```python
from build123d import *

# Parameters (mm, degrees)
SKETCH1_R                    = 211.670411635
SKETCH1_R_2                  = 6.985
SKETCH1_R_3                  = 6.6294
SKETCH1_R_4                  = 5.8928
SKETCH1_R_5                  = 4.2291
SKETCH1_R_6                  = 5.461
SKETCH1_R_7                  = 5.7531
SKETCH1_R_8                  = 5.4991
SKETCH1_R_9                  = 7.7978
SKETCH1_R_10                 = 6.6421
SKETCH1_R_11                 = 4.6228
SKETCH1_R_12                 = 5.9182
BOSS_EXTRUDE1_DEPTH          = 6
SKETCH2_R                    = 87.5
CUT_EXTRUDE1_DEPTH           = 300.4072917
F_3_8_0_375_DIAMETER_HOLE1_D = 9.525
CIRPATTERN1_COUNT            = 4


with BuildPart() as part:
    # Sketch1 → Boss-Extrude1 (new body)
    with BuildSketch(Plane.XY):
        Circle(SKETCH1_R)
        with Locations((160.80232, -67.72402)):
            Circle(SKETCH1_R_2, mode=Mode.SUBTRACT)
        with Locations((129.93116, -131.74726)):
            Circle(SKETCH1_R_3, mode=Mode.SUBTRACT)
        with Locations((88.98382, -143.60906)):
            Circle(SKETCH1_R_4, mode=Mode.SUBTRACT)
        with Locations((51.13274, -156.81706)):
            Circle(SKETCH1_R_5, mode=Mode.SUBTRACT)
        with Locations((-44.93006, -170.61434)):
            Circle(SKETCH1_R_6, mode=Mode.SUBTRACT)
        with Locations((-97.40392, -154.3431)):
            Circle(SKETCH1_R_7, mode=Mode.SUBTRACT)
        with Locations((-174.33036, -9.32688)):
            Circle(SKETCH1_R_3, mode=Mode.SUBTRACT)
        with Locations((-176.0118908, 29.95676)):
            Circle(SKETCH1_R_8, mode=Mode.SUBTRACT)
        with Locations((-89.03716, 143.4338)):
            Circle(SKETCH1_R_9, mode=Mode.SUBTRACT)
        with Locations((-26.09596, 188.2775)):
            Circle(SKETCH1_R_10, mode=Mode.SUBTRACT)
        with Locations((8.42772, 182.19674)):
            Circle(SKETCH1_R_11, mode=Mode.SUBTRACT)
        with Locations((85.42274, 152.58034)):
            Circle(SKETCH1_R_10, mode=Mode.SUBTRACT)
        with Locations((123.8123, 126.18466)):
            Circle(SKETCH1_R_12, mode=Mode.SUBTRACT)
        with Locations((169.7101, 41.9354)):
            Circle(SKETCH1_R_10, mode=Mode.SUBTRACT)
        with Locations((-115.69192, 121.86666)):
            Circle(SKETCH1_R_8, mode=Mode.SUBTRACT)
    extrude(amount=BOSS_EXTRUDE1_DEPTH)

    # Sketch2 → Cut-Extrude1 (cut, through all)
    with BuildSketch(Plane.XY.offset(6)):
        Circle(SKETCH2_R)
    extrude(amount=-CUT_EXTRUDE1_DEPTH, mode=Mode.SUBTRACT)

    # 3/8 (0.375) Diameter Hole1 (through all)
    with Locations(Plane(origin=(0, 106.68, 6), x_dir=(1, 0, 0), z_dir=(0, 0, 1))):
        with Locations((0, 0), (75.434151417, -31.245848583)):
            f_3_8_0_375_diameter_hole1 = Hole(F_3_8_0_375_DIAMETER_HOLE1_D / 2)

    # CirPattern1: 3/8 (0.375) Diameter Hole1 ×4 about axis
    cirpattern1_axis = Axis((0, 0, 0), (0, 0, 1))
    for i in range(1, CIRPATTERN1_COUNT):
        add(f_3_8_0_375_diameter_hole1.rotate(cirpattern1_axis, i * 360 / CIRPATTERN1_COUNT), mode=Mode.SUBTRACT)


solid = part.part
```
Geometry check sheet. Reference: the model listing, model coordinates, mm. Coordinates: 2 decimals unless noted, no trailing zeros. Loops run counter-clockwise (first coordinate to the right, second up) from the corner with the lowest first, then second, coordinate; pieces in that order, holes last.
Item 1: Sectioned sample at B-B, the plane y = -35.5. Record the boundary of the cut face in (x, z) (3 decimals).
Item 2: Sectioned sample at C-C, the plane z = 1.3. Count the separate pieces of the cut face and the enclosed holes in it, then the cut area to 3 significant figures.
Item 3: Thickness scan on line 1 (X direction, y = 45, z = 5.15); line 2 (Y direction, x = -43, z = 0.6); line 3 (X direction, y = -68.5, z = 5.7). Record the ranges inside material, lowest first.
Item 4: Release check for a two-part mould opening along X. For faces 1 (the face through (-167.974, -128.798, 2.958)), 2 (the face through (0.62, 111.4, 2.96)), 3 (the face through (91, 3, 6)) record: released by +X, released by -X, zero draft, split by the parting line, or undercut.
Item 5: Go/stop test with flat-tipped pins: pin 1 Ø6.5 at (x, y) = (-44.93, -170.61) entering from -Z; pin 2 Ø2 at (x, z) = (111, 4) entering from -Y; pin 3 Ø2 at (y, z) = (98, 5) entering from -X; pin 4 Ø1.5 at (y, z) = (-30, 2.5) entering from +X. Record where each tip stops, or that it passes through.
Item 6: Sectioned sample at A-A, the plane x = 25. Record the boundary of the cut face in (y, z).
Check result:
1. outline: (-208.672, 0) - (-79.975, 0) - (-79.975, 6) - (-208.672, 6) - close; (79.975, 0) - (208.672, 0) - (208.672, 6) - (79.975, 6) - close
2. separate pieces: 1
2. enclosed holes: 24
2. area: 114,000 mm2
3. line 1: x = -206.83 to -75.04, 75.04 to 163.82, 175.6 to 206.83
3. line 2: y = -207.26 to -175.72, -165.51 to -76.21, 76.21 to 207.26
3. line 3: x = -200.28 to -54.44, 54.44 to 153.86, 167.74 to 200.28
4. face 1: split by the parting line
4. face 2: undercut
4. face 3: zero draft
5. pin 1: passes through
5. pin 2: stops at y = -180.84
5. pin 3: stops at x = -188.14
5. pin 4: stops at x = 209.64
6. outline: (-210.19, 0) - (-83.85, 0) - (-83.85, 6) - (-210.19, 6) - close; (83.85, 0) - (210.19, 0) - (210.19, 6) - (83.85, 6) - close
